Part model, mm, in its own coordinate system. Face numbers are marked on the shaded views. A direction names the side the tool comes from. Round coordinates to 2 decimals unless told otherwise and drop trailing zeros. Loops run counter-clockwise (first coordinate to the right, second up) from the corner with the lowest first, then second, coordinate; pieces in that order, holes last. Notation, with made-up numbers: M 39.5,3 L 63.5,3 A21 ccw 63.5,8 Z; hole C -33,19 d10. An arc over 180 degrees is marked long. Answer as CSV lines item,"result". Start each with the question number.
Item 1: Drop flat-ended pins along their axis: pin 1 Ø2 at (x, z) = (-1.5, 1) entering from -Y; pin 2 Ø1.9 at (y, z) = (-20.5, -1) entering from -X. Give the stop position or say it passes through.
Item 2: Which spindle directions (+Z, -Z, +X, -X, +Y, -Y) get a long thin tool onto all of the face, cutting with end or side? Do the marked faces 5 and 6. Say none if no direction does.
Item 3: Band-saw the part on B-B (z = -1). Give the cut face in (x, y).
Item 4: Band-saw the part on A-A (y = -26). Give the cut face in (x, z) (3 decimals).
Item 5: Band-saw the part on D-D (x = 7.5). Give the cut face in (y, z) (3 decimals).
Item 6: Mould opens along Y. For the marked faces 1, 2, 3 and 4 say: pulls with the +Y half, pulls with the -Y half, needs draft (parallel to the pull), parting line crosses it, or undercut.
Item 7: Wall check: line 1 (X direction, y = 9, z = 2.75); line 2 (X direction, y = -22.5, z = 0.25); line 3 (Y direction, x = -1, z = -2.5). Give the ranges that are in metal, low to high.
Item 8: Band-saw the part on C-C (y = -20). Give the cut face in (x, z), and give its area (3 significant figures).
```python
from build123d import *

# Parameters (mm, degrees)
F1_DEPTH    = 3.175
F2_W        = 9.525
F2_H        = 1.4478
F3_DEPTH    = 25.4
F4_R        = 15.7740752149
F4_R_2      = 2.9681243023
F4_R_3      = 1.3729847112
F5_DEPTH    = 1.27
F6_T1_DEPTH = 31.75
F6_T3_DEPTH = 27.3506510316
F7_R        = 1.27


# Not quite as in the source:
# - a fillet or chamfer that OpenCascade refuses, or shapes differently, is made with other operations: its cross-section is extruded or revolved along the edge and cut away or added


with BuildPart() as f1:
    # F0 (on Top) → F1 (new body, symmetric)
    with BuildSketch(Plane.XY):
        Polygon((17.7787664203, 21.9838270611), (-17.1462335797, 21.9838270611), (-17.1462335797, -12.9411729389), (-14.9237335797, -12.9411729389), (-14.9237335797, -28.8161729389), (-3.4937335797, -28.8161729389), (-3.4937335797, -12.9411729389), (4.1262664203, -12.9411729389), (4.1262664203, -28.8161729389), (15.5562664203, -28.8161729389), (15.5562664203, -12.9411729389), (17.7787664203, -12.9411729389), align=None)
    extrude(amount=F1_DEPTH, both=True)

    # F2 (on Right) → F3 (cut, symmetric)
    with BuildSketch(Plane.YZ):
        with Locations((-19.2911729389, -2.4511)):
            Rectangle(F2_W, F2_H)
        with Locations((-19.2911729389, 2.4511)):
            Rectangle(F2_W, F2_H)
    extrude(amount=F3_DEPTH, both=True, mode=Mode.SUBTRACT)

    # F4 (on face) → F5 (cut)
    with BuildSketch(Plane.XY.offset(3.175)):
        with Locations((0.2568493655, 4.0185162798)):
            Circle(F4_R)
        with BuildLine():
            Line((-1.5064536128, 7.0266816765), (0.1482767001, 10.0501550651))
            ThreePointArc((0.1482767001, 10.0501550651), (0.4096706183, 7.9792062399), (1.3765677405, 6.1292695458))
            ThreePointArc((1.3765677405, 6.1292695458), (-0.1382695754, 2.1387635418), (2.9542085605, -0.8032509449))
            Line((2.9542085605, -0.8032509449), (-4.2190060268, -4.3320505521))
            Line((-4.2190060268, -4.3320505521), (-2.1576185001, -0.7580867248))
            Line((-2.1576185001, -0.7580867248), (-8.6794582017, -4.5345938661))
            Line((-8.6794582017, -4.5345938661), (-4.3788731984, 2.5767316464))
            Line((-4.3788731984, 2.5767316464), (-7.1943101482, 1.0284683409))
            Line((-7.1943101482, 1.0284683409), (-4.9999261676, 4.815935468))
            ThreePointArc((-4.9999261676, 4.815935468), (-1.6824509255, 3.4391903431), (-1.5064536128, 7.0266816765))
        make_face(mode=Mode.SUBTRACT)
        with Locations((3.6213599069, 2.9943462909)):
            Circle(F4_R_2, mode=Mode.SUBTRACT)
        with Locations((-2.8567614499, 5.2948631346)):
            Circle(F4_R_3, mode=Mode.SUBTRACT)
        with BuildLine():
            ThreePointArc((2.3814487819, 6.6452990552), (7.6456545146, 14.2492672348), (6.8950720548, 5.0314139032))
            ThreePointArc((6.8950720548, 5.0314139032), (4.9195289911, 6.6249926126), (2.3814487819, 6.6452990552))
        make_face(mode=Mode.SUBTRACT)
    extrude(amount=-F5_DEPTH, mode=Mode.SUBTRACT)

    # F6: fillet of radius 5.08 on 4 edges, made by hand

    # F6_s2 → F6_t1 (cut)
    with BuildSketch(Plane.XY.offset(-15.875)):
        with BuildLine():
            ThreePointArc((12.6987664203, 21.9838270611), (16.2908688687, 20.4959295096), (17.7787664203, 16.9038270611))
            Line((17.7787664203, 16.9038270611), (17.7787664203, 21.9838270611))
            Line((17.7787664203, 21.9838270611), (12.6987664203, 21.9838270611))
        make_face()
        with BuildLine():
            ThreePointArc((-17.1462335797, 16.9038270611), (-15.6583360282, 20.4959295096), (-12.0662335797, 21.9838270611))
            Line((-12.0662335797, 21.9838270611), (-17.1462335797, 21.9838270611))
            Line((-17.1462335797, 21.9838270611), (-17.1462335797, 16.9038270611))
        make_face()
    extrude(amount=F6_T1_DEPTH, mode=Mode.SUBTRACT)

    # F6_s4 → F6_t3 (cut)
    with BuildSketch(Plane.XY.offset(-13.6753255158)):
        with BuildLine():
            ThreePointArc((-14.9237335797, -12.9411729388), (-16.5563616403, -11.1169951731), (-17.1462335797, -8.7410427325))
            Line((-17.1462335797, -8.7410427325), (-17.1462335797, -12.9411729389))
            Line((-17.1462335797, -12.9411729389), (-14.9237335797, -12.9411729388))
        make_face()
        with BuildLine():
            ThreePointArc((17.7787664203, -8.7410427325), (17.1888944808, -11.1169951731), (15.5562664203, -12.9411729388))
            Line((15.5562664203, -12.9411729388), (17.7787664203, -12.9411729389))
            Line((17.7787664203, -12.9411729389), (17.7787664203, -8.7410427325))
        make_face()
    extrude(amount=F6_T3_DEPTH, mode=Mode.SUBTRACT)

    # F7
    f7_edges = [f1.edges().sort_by_distance(p)[0] for p in [
        (-14.923734, -14.528673, 2.4511),
        (-3.493734, -14.528673, 2.4511),
        (15.556266, -14.528673, 2.4511),
        (4.126266, -14.528673, 2.4511),
        (15.556266, -14.528673, -2.4511),
        (4.126266, -14.528673, -2.4511),
        (-14.923734, -14.528673, -2.4511),
        (-3.493734, -14.528673, -2.4511),
        (-3.493734, -24.053673, -2.4511),
        (-3.493734, -24.053673, 2.4511),
        (15.556266, -24.053673, -2.4511),
        (15.556266, -24.053673, 2.4511),
        (15.556266, -28.816173, 0),
        (4.126266, -28.816173, 0),
        (-3.493734, -28.816173, 0),
        (-14.923734, -28.816173, 0),
        (-14.923734, -24.053673, 2.4511),
        (-14.923734, -24.053673, -2.4511),
        (4.126266, -24.053673, 2.4511),
        (4.126266, -24.053673, -2.4511),
    ]]
    fillet(f7_edges, radius=F7_R)


solid = f1.part
```
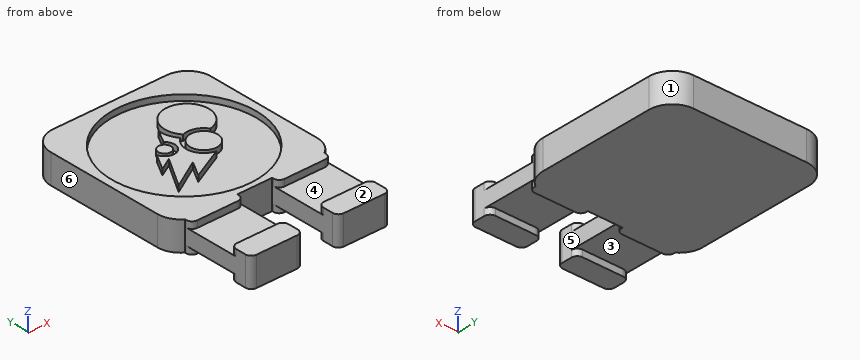
Answer block:
1,pin 1,"stops at y = -12.94"
1,pin 2,"stops at x = -14.92"
2,face 5,"+Z, -Z, -Y"
2,face 6,"+Z, -Z, -X, +Y, -Y"
3,outline,"M -17.15,-8.74 A5.08 ccw -14.92,-12.94 L -14.92,-27.55 A1.27 ccw -13.65,-28.82 L -4.76,-28.82 A1.27 ccw -3.49,-27.55 L -3.49,-12.94 L 4.13,-12.94 L 4.13,-27.55 A1.27 ccw 5.4,-28.82 L 14.29,-28.82 A1.27 ccw 15.56,-27.55 L 15.56,-12.94 A5.08 ccw 17.78,-8.74 L 17.78,16.9 A5.08 ccw 12.7,21.98 L -12.07,21.98 A5.08 ccw -17.15,16.9 Z"
4,outline,"M -14.924,-3.175 L -3.494,-3.175 L -3.494,3.175 L -14.924,3.175 Z; M 4.126,-3.175 L 15.556,-3.175 L 15.556,3.175 L 4.126,3.175 Z"
5,outline,"M -28.816,-3.175 L -24.054,-3.175 L -24.054,-1.727 L -14.529,-1.727 L -14.529,-3.175 L 21.984,-3.175 L 21.984,3.175 L 18.031,3.175 L 18.031,1.905 L 14.299,1.905 L 14.299,3.175 L 5.183,3.175 L 5.183,1.905 L -9.994,1.905 L -9.994,3.175 L -14.529,3.175 L -14.529,1.727 L -24.054,1.727 L -24.054,3.175 L -28.816,3.175 Z"
6,face 1,"pulls with the +Y half"
6,face 2,"needs draft"
6,face 3,"undercut"
6,face 4,"undercut"
7,line 1,"x = -17.15 to -14.71, -0.43 to 0.19, 1.3 to 10.76, 15.22 to 17.78"
7,line 2,"x = -14.92 to -3.49, 4.13 to 15.56"
7,line 3,"y = -12.94 to 21.98"
8,outline,"M -14.92,-1.73 L -3.49,-1.73 L -3.49,1.73 L -14.92,1.73 Z; M 4.13,-1.73 L 15.56,-1.73 L 15.56,1.73 L 4.13,1.73 Z"
8,area,"79.0 mm^2"
